from build123d import *

# Parameters (mm, degrees)
SALIENTE_EXTRUIR1_DEPTH      = 0.25
SALIENTE_EXTRUIR1_DEPTH_BACK = 0.25
CROQUIS2_R                   = 1
SALIENTE_EXTRUIR2_DEPTH      = 5


with BuildPart() as part:
    # Croquis1 → Saliente-Extruir1 (new, two sides: drawn at the far end of the back side and taken through both)
    with BuildSketch(Plane(origin=(0, 0, 0), x_dir=(1, 0, 0), z_dir=(0, 1, 0)).offset(-SALIENTE_EXTRUIR1_DEPTH_BACK)):
        with BuildLine():
            Line((8, 0), (3.5, 0))
            ThreePointArc((3.5, 0), (2.249756634, 2.681155551), (-0.607768622, 3.446827136))
            Line((-0.607768622, 3.446827136), (-1.389185421, 7.878462024))
            ThreePointArc((-1.389185421, 7.878462024), (-6.128355545, 5.142300877), (-8, 0))
            Line((-8, 0), (-3.5, 0))
            ThreePointArc((-3.5, 0), (-2.249756634, -2.681155551), (0.607768622, -3.446827136))
            Line((0.607768622, -3.446827136), (1.389185421, -7.878462024))
            ThreePointArc((1.389185421, -7.878462024), (6.128355545, -5.142300877), (8, 0))
        make_face()
    extrude(amount=SALIENTE_EXTRUIR1_DEPTH + SALIENTE_EXTRUIR1_DEPTH_BACK)

    # Croquis2 → Saliente-Extruir2 (add)
    with BuildSketch(Plane(origin=(0, 0.25, 0), x_dir=(1, 0, 0), z_dir=(0, 1, 0))):
        with Locations(Location((0, 0, 0), (0, 0, 270))):
            Circle(CROQUIS2_R)
    extrude(amount=SALIENTE_EXTRUIR2_DEPTH)


solid = part.part
Geometry: final body of the model. Coordinates: model frame, mm. A direction names the side the tool comes from. Round coordinates to 2 decimals unless told otherwise and drop trailing zeros. Loops run counter-clockwise (first coordinate to the right, second up) from the corner with the lowest first, then second, coordinate; pieces in that order, holes last.
Q1. Section A-A on x = 0. Return loops of the section in (y, z).
Q2. Section C-C on y = 2.65. Return loops of the section in (x, z), plus the area to 3 significant figures.
Q3. Section B-B on z = 0.25. Return loops of the section in (x, y).
Q4. Section D-D on z = -7. Return loops of the section in (x, y), plus the area to 3 significant figures.
Q5. Material intervals for L1, parallel to Y at x = -3.25, z = -1.75; L2, parallel to X at y = 0.2, z = -5 (3 decimals); L3, parallel to Z at x = 1.5, y = 0.2, sorted ascending.
Q6. Pin query (flat end, axial travel): P1, Ø2, axis at x = -2.5, z = 2.5, coming from the -Y side; P2, Ø2, axis at y = 3.5, z = 0, coming from the -X side; P3, Ø3, axis at y = 0.5, z = 6, coming from the +X side. Return the tip coordinate at first contact, or that it passes through.
Q7. Access query for faces 1 (the cylindrical face through (6.08, 0, 5.2)), 2 (the cylindrical face through (-1, 3, 0)). Directions: +Z, -Z, +X, -X, +Y, -Y. A direction counts if a zero-diameter tool reaches every point of the face in a straight line with its end or side. Return the directions, or none.
Evaluation:
1. outline: (-0.25, -3.5) - (0.25, -3.5) - (0.25, -1) - (5.25, -1) - (5.25, 1) - (0.25, 1) - (0.25, 3.5) - (-0.25, 3.5) - close
2. outline: circle Ø2 at (0, 0)
2. area: 3.14 mm2
3. outline: (-3.49, -0.25) - (8, -0.25) - (8, 0.25) - (0.97, 0.25) - (0.97, 5.25) - (-0.97, 5.25) - (-0.97, 0.25) - (-3.49, 0.25) - close
4. outline: (-3.87, -0.25) - (-1.23, -0.25) - (-1.23, 0.25) - (-3.87, 0.25) - close
4. area: 1.32 mm2
5. L1: y = -0.25 to 0.25
5. L2: x = -6.245 to -0.882
5. L3: z = -3.16 to 7.86
6. P1: stops at y = -0.25
6. P2: stops at x = -1
6. P3: stops at x = 6.6
7. face 1: +Z, +X, +Y, -Y
7. face 2: +Y
